For this review, take the finished solid that the model builds, in its own axes (mm). Round coordinates to 2 decimals unless told otherwise and drop trailing zeros. Order: outer loops, then holes, each group sorted by start corner. A loop starts at its lowest first (then second) coordinate and runs counter-clockwise, first axis right, second up. Notation, with made-up numbers: (22.25, -18.75) - (57.25, -18.75) arc R8 ccw to (57.25, -10.75) - close; hole circle Ø1 at (-11, 27). An arc over 180 degrees is marked (long way). One line per item, written item: value.
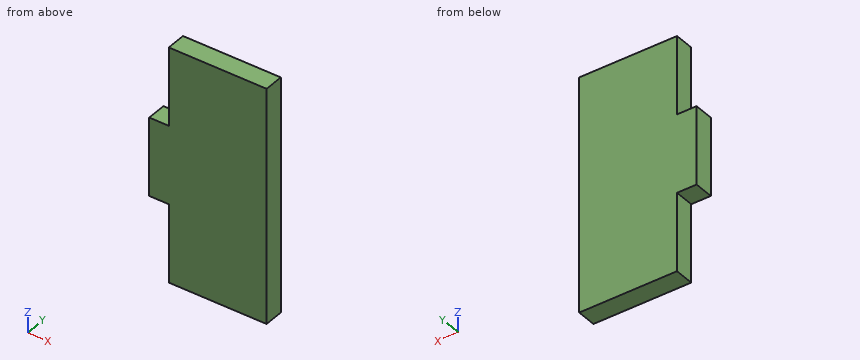
```python
from build123d import *

# Parameters (mm, degrees)
F0_W     = 3.175
F0_H     = 12.7
F1_DEPTH = 3.175


with BuildPart() as f1:
    # F0 (on Front) → F1 (new body)
    with BuildSketch(Plane.XZ):
        with Locations((-7.9375, 0)):
            Rectangle(F0_W, F0_H)
        Polygon((9.525, -19.05), (9.525, 19.05), (-6.35, 19.05), (-6.35, 6.35), (-6.35, -6.35), (-6.35, -19.05), align=None)
    extrude(amount=F1_DEPTH)


solid = f1.part
```
Item 1: Take a section at A-A (y = -2.7). Write out the cut boundary in (x, z) (3 decimals).
Returned:
outline: (-9.525, -6.35) - (-6.35, -6.35) - (-6.35, -19.05) - (9.525, -19.05) - (9.525, 19.05) - (-6.35, 19.05) - (-6.35, 6.35) - (-9.525, 6.35) - close
Item 2: Take a section at B-B (z = -12). Write out the cut boundary in (x, y) (3 decimals).
Returned:
outline: (-6.35, -3.175) - (9.525, -3.175) - (9.525, 0) - (-6.35, 0) - close
Item 3: For P1, Ø1.6, axis at x = -8.5, y = -1, coming from the +Z side; P2, Ø1.6, axis at x = -8.5, y = -1.5, coming from the -Z side; P3, Ø8, axis at x = -6.5, z = -11.5, coming from the -Y side (3 decimals), all flat-tipped, find the tip position at first contact; note any pin that passes through.
Returned:
P1: z = 6.35
P2: z = -6.35
P3: y = -3.175
Item 4: Wall thickness on line 1 (X direction, y = -2.9, z = 7) (3 decimals): over which ranges is the line inside the solid? List them lowest first.
Returned:
line 1: -6.35 to 9.525
